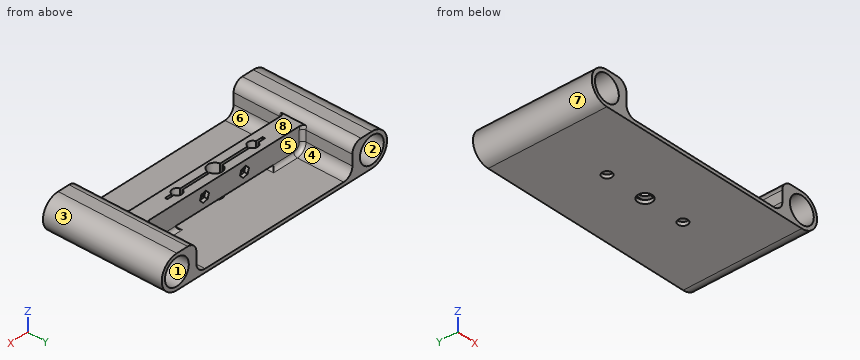
from build123d import *

# Parameters (mm, degrees)
SKETCH1_R                    = 11
BOSS_EXTRUDE1_DEPTH          = 100
FILLET1_R                    = 8
SKETCH2_R                    = 4.1
SKETCH2_R_2                  = 6
CUT_EXTRUDE1_DEPTH           = 10
BOSS_EXTRUDE2_START          = 20
SKETCH3_R                    = 4.1
SKETCH3_R_2                  = 6
BOSS_EXTRUDE2_DEPTH          = 20
FILLET2_R                    = 3
CUT_EXTRUDE_THIN1_DEPTH      = 183.94618817
CUT_EXTRUDE_THIN1_DEPTH_BACK = 20
CUT_EXTRUDE_THIN2_DEPTH      = 163.832913644
CUT_EXTRUDE_THIN2_DEPTH_BACK = 20
FILLET3_R                    = 3
CUT_EXTRUDE2_DEPTH           = 161.472919104
CUT_EXTRUDE2_DEPTH_BACK      = 161.472919104
SKETCH6_R                    = 2.25
CUT_EXTRUDE3_DEPTH           = 3


with BuildPart() as part:
    # Sketch1 → Boss-Extrude1 (new body)
    with BuildSketch(Plane(origin=(0, 0, 0), x_dir=(1, 0, 0), z_dir=(0, 1, 0))):
        with BuildLine():
            Line((137.460581558, -14.5), (119.460581558, -14.5))
            Line((119.460581558, -14.5), (119.460581558, 10.5))
            Line((119.460581558, 10.5), (-24.539418442, 10.5))
            Line((-24.539418442, 10.5), (-24.539418442, -14.5))
            Line((-24.539418442, -14.5), (-42.539418442, -14.5))
            ThreePointArc((-42.539418442, -14.5), (-56.539418442, -0.5), (-42.539418442, 13.5))
            Line((-42.539418442, 13.5), (137.460581558, 13.5))
            ThreePointArc((137.460581558, 13.5), (151.460581558, -0.5), (137.460581558, -14.5))
        make_face()
        with Locations(Location((-42.539418442, -0.5, 0), (0, 0, 270))):
            Circle(SKETCH1_R, mode=Mode.SUBTRACT)
        with Locations(Location((137.460581558, -0.5, 0), (0, 0, 270))):
            Circle(SKETCH1_R, mode=Mode.SUBTRACT)
    extrude(amount=BOSS_EXTRUDE1_DEPTH)

    # Fillet1
    fillet1_edges = [part.edges().sort_by_distance(p)[0] for p in [
        (119.460581558, 50, 14.5),
        (119.460581558, 50, -10.5),
        (-24.539418442, 50, -10.5),
        (-24.539418442, 50, 14.5),
    ]]
    fillet(fillet1_edges, radius=FILLET1_R)

    # Sketch2 → Cut-Extrude1 (cut)
    with BuildSketch(Plane.XY.offset(-10.5)):
        with Locations((12.460581558, 50)):
            Circle(SKETCH2_R)
        with Locations((82.460581558, 50)):
            Circle(SKETCH2_R)
        with Locations((47.460581558, 50)):
            Circle(SKETCH2_R_2)
    extrude(amount=-CUT_EXTRUDE1_DEPTH, mode=Mode.SUBTRACT)

    # Sketch3 → Boss-Extrude2 (add)
    with BuildSketch(Plane.XY.offset(-10.5).offset(BOSS_EXTRUDE2_START)):
        Polygon((12.460581558, 58), (82.460581558, 58), (124.149440998, 58), (124.149440998, 42), (82.460581558, 42), (12.460581558, 42), (-28.8662965, 42), (-28.8662965, 58), (-16.539418442, 58), align=None)
        with Locations((12.460581558, 50)):
            Circle(SKETCH3_R, mode=Mode.SUBTRACT)
        with Locations((82.460581558, 50)):
            Circle(SKETCH3_R, mode=Mode.SUBTRACT)
        with Locations((47.460581558, 50)):
            Circle(SKETCH3_R_2, mode=Mode.SUBTRACT)
    extrude(amount=-BOSS_EXTRUDE2_DEPTH)

    # Fillet2
    fillet2_edges = [part.edges().sort_by_distance(p)[0] for p in [
        (-24.686725022, 58, 8.0281381),
        (-24.686725022, 42, 8.0281381),
        (47.460581558, 42, -10.5),
        (117.117435807, 42, -8.156854249),
        (119.460581558, 42, 2),
        (-24.539418442, 42, 2),
        (-22.196272692, 42, -8.156854249),
        (119.607888138, 42, 8.0281381),
        (119.460581558, 58, 2),
        (117.117435807, 58, -8.156854249),
        (47.460581558, 58, -10.5),
        (-22.196272692, 58, -8.156854249),
        (-24.539418442, 58, 2),
        (119.607888138, 58, 8.0281381),
    ]]
    fillet(fillet2_edges, radius=FILLET2_R)

    # Sketch4 → Cut-Extrude-Thin1 (cut, two sides: drawn at the far end of the back side and taken through both)
    with BuildSketch(Plane.XY.offset(9.5).offset(-CUT_EXTRUDE_THIN1_DEPTH_BACK)):
        Polygon((92.460581558, 51), (47.460581558, 51), (2.460581558, 51), (2.460581558, 49), (47.460581558, 49), (92.460581558, 49), align=None)
    extrude(amount=CUT_EXTRUDE_THIN1_DEPTH + CUT_EXTRUDE_THIN1_DEPTH_BACK, mode=Mode.SUBTRACT)

    # Sketch5 → Cut-Extrude-Thin2 (cut, two sides: drawn at the far end of the back side and taken through both)
    with BuildSketch(Plane(origin=(0, 42, 0), x_dir=(-1, 0, 0), z_dir=(0, -1, 0)).offset(-CUT_EXTRUDE_THIN2_DEPTH_BACK)):
        Polygon((-2.460581558, 7.5), (-47.460581558, 7.5), (-92.460581558, 7.5), (-92.460581558, 10.5), (-47.460581558, 10.5), (-2.460581558, 10.5), align=None)
    extrude(amount=CUT_EXTRUDE_THIN2_DEPTH + CUT_EXTRUDE_THIN2_DEPTH_BACK, mode=Mode.SUBTRACT)

    # Fillet3
    fillet3_edges = [part.edges().sort_by_distance(p)[0] for p in [
        (2.460581558, 50, -10.5),
        (92.460581558, 50, -10.5),
    ]]
    fillet(fillet3_edges, radius=FILLET3_R - 0.0001)  # a hair under: the kernel refuses the full size

    # Sketch6 → Cut-Extrude2 (cut, two sides: drawn at the far end of the back side and taken through both)
    with BuildSketch(Plane(origin=(0, 49, 0), x_dir=(1, 0, 0), z_dir=(0, 1, 0)).offset(-CUT_EXTRUDE2_DEPTH_BACK)):
        with Locations(Location((28.990631201, -1, 0), (0, 0, 270))):
            Circle(SKETCH6_R)
        with Locations(Location((65.930531914, -1, 0), (0, 0, 270))):
            Circle(SKETCH6_R)
    extrude(amount=CUT_EXTRUDE2_DEPTH + CUT_EXTRUDE2_DEPTH_BACK, mode=Mode.SUBTRACT)

    # Sketch7 → Cut-Extrude3 (cut)
    with BuildSketch(Plane(origin=(0, 58, 0), x_dir=(1, 0, 0), z_dir=(0, 1, 0))):
        Polygon((33.150591825, -0.026315789), (30.227376252, 3.089473684), (26.067415628, 2.115789474), (24.830670578, -1.973684211), (27.753886151, -5.089473684), (31.913846775, -4.115789474), align=None)
        Polygon((70.090492538, -0.026315789), (67.167276964, 3.089473684), (63.007316341, 2.115789474), (61.77057129, -1.973684211), (64.693786864, -5.089473684), (68.853747488, -4.115789474), align=None)
    extrude(amount=-CUT_EXTRUDE3_DEPTH, mode=Mode.SUBTRACT)


solid = part.part
Design review of the part built by this model. Coordinates are the model's own, in mm. Face numbers are marked on the shaded views. A direction names the side the tool comes from. Round coordinates to 2 decimals unless told otherwise and drop trailing zeros. Write each loop counter-clockwise with the first axis right and the second up, starting at its lowest first coordinate (ties: lowest second). Pieces come first, ordered by that corner, then holes. Notation, with made-up numbers: (-15.5, 86) - (-5.5, 86) arc R19 ccw to (-5.5, 102) - close; hole circle Ø8 at (-14, 2.25). An arc over 180 degrees is marked (long way). Return JSON: item names as keys, results as strings. Group by question number.
Item 1: We need section A-A on x = 18.5. Write out the cut boundary in (y, z).
Item 2: We need section C-C on x = -9. Write out the cut boundary in (y, z), and give its area (3 significant figures).
Item 3: For probe 1 along X at (y, z) = (28, 1.5); probe 2 along Z at (x, y) = (69, 43.5); probe 3 along Z at (x, y) = (137.5, 86.5), list the stretches that pass through material, from the lowest coordinate up. Write a range as [from, to].
Item 4: The part is to be moulded in two halves that separate along Z. For the marked faces 1, 2, 3 and 4, say which applies: pulls with the +Z half, pulls with the -Z half, needs draft (parallel to the pull), parting line crosses it, or undercut.
Item 5: Machinability: for the marked faces 5, 6, 7 and 8, which of the approach directions +Z, -Z, +X, -X, +Y, -Y give a long, thin tool a straight path to every point of the face, cutting with its end or side? Answer none if there is none.
Item 6: We need section B-B on y = 64.5. Write out the cut boundary in (x, z).
Item 7: Insertion check: P1, Ø4.5, axis at y = 74.5, z = 2.5, coming from the +X side; P2, Ø13.5, axis at x = 61.5, z = 2, coming from the +Y side; P3, Ø2, axis at y = 23.5, z = 11.5, coming from the -X side; P4, Ø6, axis at x = 28.99, z = 1, coming from the -Y side. Each pin has a flat end and moves straight along its axis. Give the tip position at first contact, or say it passes through.
Model answer:
{
 "1": {"outline": "(0, -13.5) - (100, -13.5) - (100, -10.5) - (0, -10.5) - close; (42, -7.5) - (49, -7.5) - (49, 9.5) - (42, 9.5) - close; (51, -7.5) - (58, -7.5) - (58, 9.5) - (51, 9.5) - close"},
 "2": {"outline": "(0, -13.5) - (100, -13.5) - (100, -10.5) - (61, -10.5) arc R3 cw to (58, -7.5) - (58, 9.5) - (42, 9.5) - (42, -7.5) arc R3 cw to (39, -10.5) - (0, -10.5) - close", "area": "624 mm²"},
 "3": {"probe 1": "x = [-56.5, -53.49], [-31.58, -24.54], [119.46, 126.51], [148.42, 151.42]", "probe 2": "z = [-13.5, -10.5], [-7.5, 9.5]", "probe 3": "z = [-13.5, -10.5], [11.5, 14.5]"},
 "4": {"face 1": "undercut", "face 2": "undercut", "face 3": "parting line crosses it", "face 4": "pulls with the +Z half"},
 "5": {"face 5": "+Z, +Y", "face 6": "+Z, -Y", "face 7": "-X, +Y, -Y", "face 8": "+Z, +Y, -Y"},
 "6": {"outline": "(-42.54, -13.5) - (137.46, -13.5) arc R14 ccw to (137.46, 14.5) - (127.46, 14.5) arc R8 ccw to (119.46, 6.5) - (119.46, -2.5) arc R8 cw to (111.46, -10.5) - (-16.54, -10.5) arc R8 cw to (-24.54, -2.5) - (-24.54, 6.5) arc R8 ccw to (-32.54, 14.5) - (-42.54, 14.5) arc R14 ccw to start; hole circle Ø22 at (-42.54, 0.5); hole circle Ø22 at (137.46, 0.5)"},
 "7": {"P1": "stops at x = 151.46", "P2": "stops at y = 58", "P3": "stops at x = -52.34", "P4": "stops at y = 42"}
}
